Geometry check sheet. Reference: the model listing, model coordinates, mm. Face numbers are marked on the shaded views. A direction names the side the tool comes from. Give positions to 0.01 mm unless a question says otherwise; leave off trailing zeros. Order: outer loops, then holes, each group sorted by start corner. A loop starts at its lowest first (then second) coordinate and runs counter-clockwise, first axis right, second up. Notation, with made-up numbers: M 10.25,33 L 55.25,33 A31 ccw 55.25,64 Z; hole C 68,-20 d10. An arc over 180 degrees is marked long. Answer as CSV lines item,"result". Start each with the question number.
```python
from build123d import *

# Parameters (mm, degrees)
CYLINDER009_R          = 1.1
CYLINDER009_DEPTH      = 10
CYLINDER008_W          = 7
CYLINDER008_H          = 10
CYLINDER008_ANGLE      = 133
BOX008_W               = 4.5
BOX008_H               = 3.6
BOX008_DEPTH           = 10
BOX009_W               = 4.5
BOX009_H               = 3.6
BOX009_DEPTH           = 10
BOX005_W               = 3.4
BOX005_H               = 2.7
BOX005_DEPTH           = 3.5
BOX005_PLACEMENT_ANGLE = 50
BOX006_W               = 4
BOX006_H               = 2.7
BOX006_DEPTH           = 3.5
BOX006_PLACEMENT_ANGLE = 40
BOX004_W               = 3
BOX004_H               = 3
BOX004_DEPTH           = 3.5
BOX004_PLACEMENT_ANGLE = 220
BOX003_W               = 3
BOX003_H               = 3
BOX003_DEPTH           = 3.5
BOX003_PLACEMENT_ANGLE = 220
BOX001_W               = 3.4
BOX001_H               = 2.7
BOX001_DEPTH           = 3.5
BOX001_PLACEMENT_ANGLE = 50
BOX002_W               = 4
BOX002_H               = 2.7
BOX002_DEPTH           = 3.5
BOX002_PLACEMENT_ANGLE = 40
CYLINDER003_R          = 4.9
CYLINDER003_DEPTH      = 10
CYLINDER002_R          = 5.8
CYLINDER002_DEPTH      = 10
CYLINDER001_R          = 4.9
CYLINDER001_DEPTH      = 10
CYLINDER_R             = 5.7
CYLINDER_DEPTH         = 10
BOX007_W               = 38
BOX007_H               = 2
BOX007_DEPTH           = 1.5
CYLINDER004_R          = 5.95
CYLINDER004_DEPTH      = 3.5
BOX_W                  = 38
BOX_H                  = 19
BOX_DEPTH              = 2
CYLINDER005_R          = 5.95
CYLINDER005_DEPTH      = 3.5


with BuildPart() as cylinder009:
    # Cylinder009 → Cylinder009 (new body)
    with BuildSketch(Plane(origin=(13, 4.85, 0), x_dir=(1, 0, 0), z_dir=(0, 0, 1))):
        Circle(CYLINDER009_R)
    extrude(amount=CYLINDER009_DEPTH)


with BuildPart() as fusion002:
    # Cylinder008 → Cylinder008 (revolve)
    with BuildSketch(Plane(origin=(13.3, 5.5, 0), x_dir=(-1, 0, 0), z_dir=(0, 1, 0))):
        with Locations((3.5, 5)):
            Rectangle(CYLINDER008_W, CYLINDER008_H)
    revolve(axis=Axis((13.3, 5.5, 0), (0, 0, 1)), revolution_arc=CYLINDER008_ANGLE)

    # Fusion002: union Cylinder009
    add(cylinder009.part)


with BuildPart() as cube001_x_button_well_left_cutter:
    # Box008 → Box008 (new body)
    with BuildSketch(Plane(origin=(6.8, 10.2, 0.25), x_dir=(1, 0, 0), z_dir=(0, 0, 1))):
        with Locations((2.25, 1.8)):
            Rectangle(BOX008_W, BOX008_H)
    extrude(amount=BOX008_DEPTH)


with BuildPart() as cube002_y_button_well_left_cutter:
    # Box009 → Box009 (new body)
    with BuildSketch(Plane(origin=(21.1, 5.6, 0.25), x_dir=(1, 0, 0), z_dir=(0, 0, 1))):
        with Locations((2.25, 1.8)):
            Rectangle(BOX009_W, BOX009_H)
    extrude(amount=BOX009_DEPTH)


with BuildPart() as box005:
    # Box005 → Box005 (new body)
    with BuildSketch(Plane.XY):
        with Locations((1.7, 1.35)):
            Rectangle(BOX005_W, BOX005_H)
    extrude(amount=BOX005_DEPTH)


with BuildPart() as box005_1:
    # Box005 placement: moved
    add(box005.part.moved(Location((17.5, 7.5, 0.25))).rotate(Axis((17.5, 7.5, 0.25), (0, 0, -1)), BOX005_PLACEMENT_ANGLE))


with BuildPart() as box006:
    # Box006 → Box006 (new body)
    with BuildSketch(Plane.XY):
        with Locations((2, 1.35)):
            Rectangle(BOX006_W, BOX006_H)
    extrude(amount=BOX006_DEPTH)


with BuildPart() as box006_1:
    # Box006 placement: moved
    add(box006.part.moved(Location((33.7, 9, 0.25))).rotate(Axis((33.7, 9, 0.25), (0, 0, 1)), BOX006_PLACEMENT_ANGLE))


with BuildPart() as cube001_a_button_well_cutter:
    # Box004 → Box004 (new body)
    with BuildSketch(Plane.XY):
        with Locations((1.5, 1.5)):
            Rectangle(BOX004_W, BOX004_H)
    extrude(amount=BOX004_DEPTH)


with BuildPart() as cube001_a_button_well_cutter_1:
    # Box004 placement: moved
    add(cube001_a_button_well_cutter.part.moved(Location((9.8, 9.4, 0.25))).rotate(Axis((9.8, 9.4, 0.25), (0, 0, 1)), BOX004_PLACEMENT_ANGLE))


with BuildPart() as cube001_b_button_well_cutter:
    # Box003 → Box003 (new body)
    with BuildSketch(Plane.XY):
        with Locations((1.5, 1.5)):
            Rectangle(BOX003_W, BOX003_H)
    extrude(amount=BOX003_DEPTH)


with BuildPart() as cube001_b_button_well_cutter_1:
    # Box003 placement: moved
    add(cube001_b_button_well_cutter.part.moved(Location((23.5, 5, 0.25))).rotate(Axis((23.5, 5, 0.25), (0, 0, 1)), BOX003_PLACEMENT_ANGLE))


with BuildPart() as box001:
    # Box001 → Box001 (new body)
    with BuildSketch(Plane.XY):
        with Locations((1.7, 1.35)):
            Rectangle(BOX001_W, BOX001_H)
    extrude(amount=BOX001_DEPTH)


with BuildPart() as box001_1:
    # Box001 placement: moved
    add(box001.part.moved(Location((31.5, 2.9, 0.25))).rotate(Axis((31.5, 2.9, 0.25), (0, 0, -1)), BOX001_PLACEMENT_ANGLE))


with BuildPart() as cube001_y_button_well_right_top_cutter:
    # Box002 → Box002 (new body)
    with BuildSketch(Plane.XY):
        with Locations((2, 1.35)):
            Rectangle(BOX002_W, BOX002_H)
    extrude(amount=BOX002_DEPTH)


with BuildPart() as cube001_y_button_well_right_top_cutter_1:
    # Box002 placement: moved
    add(cube001_y_button_well_right_top_cutter.part.moved(Location((19.5, 13.5, 0.25))).rotate(Axis((19.5, 13.5, 0.25), (0, 0, 1)), BOX002_PLACEMENT_ANGLE))


with BuildPart() as cylinder_y_button_well_inner:
    # Cylinder003 → Cylinder003 (new body)
    with BuildSketch(Plane(origin=(29.55, 7.35, 0), x_dir=(1, 0, 0), z_dir=(0, 0, 1))):
        Circle(CYLINDER003_R)
    extrude(amount=CYLINDER003_DEPTH)


with BuildPart() as cylinder_b_button_well_inner:
    # Cylinder002 → Cylinder002 (new body)
    with BuildSketch(Plane(origin=(18.7, -1.6, 0), x_dir=(1, 0, 0), z_dir=(0, 0, 1))):
        Circle(CYLINDER002_R)
    extrude(amount=CYLINDER002_DEPTH)


with BuildPart() as cylinder_x_button_well_inner:
    # Cylinder001 → Cylinder001 (new body)
    with BuildSketch(Plane(origin=(15.55, 11.7, 0), x_dir=(1, 0, 0), z_dir=(0, 0, 1))):
        Circle(CYLINDER001_R)
    extrude(amount=CYLINDER001_DEPTH)


with BuildPart() as cylinder_a_button_well_inner:
    # Cylinder → Cylinder (new body)
    with BuildSketch(Plane(origin=(4.6, 3.2, 0), x_dir=(1, 0, 0), z_dir=(0, 0, 1))):
        Circle(CYLINDER_R)
    extrude(amount=CYLINDER_DEPTH)


with BuildPart() as fusion001:
    # Box007 → Box007 (new body)
    with BuildSketch(Plane(origin=(0, 18, 0), x_dir=(1, 0, 0), z_dir=(0, 0, 1))):
        with Locations((19, 1)):
            Rectangle(BOX007_W, BOX007_H)
    extrude(amount=BOX007_DEPTH)

    # Fusion001: union Cube001(x_button_well_left_cutter), Cube002(y_button_well_left_cutter), Box005, Box006, Cube001(a_button_well_cutter), Cube001(b_button_well_cutter), Box001, Cube001(y_button_well_right_top_cutter), Cylinder(y_button_well_inner), Cylinder(b_button_well_inner), Cylinder(x_button_well_inner), Cylinder(a_button_well_inner)
    add(cube001_x_button_well_left_cutter.part)
    add(cube002_y_button_well_left_cutter.part)
    add(box005_1.part)
    add(box006_1.part)
    add(cube001_a_button_well_cutter_1.part)
    add(cube001_b_button_well_cutter_1.part)
    add(box001_1.part)
    add(cube001_y_button_well_right_top_cutter_1.part)
    add(cylinder_y_button_well_inner.part)
    add(cylinder_b_button_well_inner.part)
    add(cylinder_x_button_well_inner.part)
    add(cylinder_a_button_well_inner.part)


with BuildPart() as cylinder_x_button_well_outer:
    # Cylinder004 → Cylinder004 (new body)
    with BuildSketch(Plane(origin=(15.55, 11.7, 0), x_dir=(1, 0, 0), z_dir=(0, 0, 1))):
        Circle(CYLINDER004_R)
    extrude(amount=CYLINDER004_DEPTH)


with BuildPart() as cube:
    # Box → Box (new body)
    with BuildSketch(Plane.XY):
        with Locations((19, 9.5)):
            Rectangle(BOX_W, BOX_H)
    extrude(amount=BOX_DEPTH)


with BuildPart() as cut001:
    # Cylinder005 → Cylinder005 (new body)
    with BuildSketch(Plane(origin=(29.55, 7.35, 0), x_dir=(1, 0, 0), z_dir=(0, 0, 1))):
        Circle(CYLINDER005_R)
    extrude(amount=CYLINDER005_DEPTH)

    # Fusion: union Cylinder(x_button_well_outer), Cube
    add(cylinder_x_button_well_outer.part)
    add(cube.part)

    # Cut: cut Fusion001
    add(fusion001.part, mode=Mode.SUBTRACT)

    # Cut001: cut Fusion002
    add(fusion002.part, mode=Mode.SUBTRACT)


solid = cut001.part
```
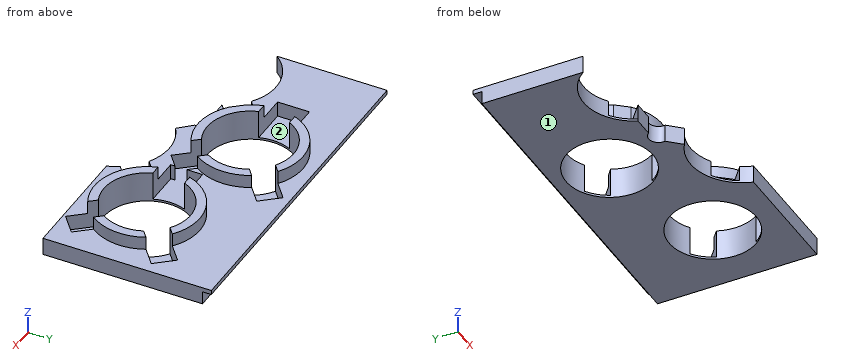
Item 1: Scan lines: line 1 along X through (y, z) = (7.35, 0.7); line 2 along X through (y, z) = (11.5, 1.65); line 3 along X through (y, z) = (5.75, 1.45). Record each from-to range of solid material in increasing order.
Item 2: Section check D-D on x = 4. Record the boundary of the cut face in (y, z).
Item 3: Section check C-C on x = 8.5. Record the boundary of the cut face in (y, z).
Item 4: Depth check by flat-ended pin: pin 1 Ø0.8 at (x, z) = (20, 1) entering from +Y; pin 2 Ø1.5 at (x, z) = (15.5, 3) entering from +Y; pin 3 Ø1.3 at (x, y) = (21.5, 6.5) entering from +Z. Enter the tip coordinate at first touch or a pass-through.
Item 5: Section check A-A on x = 29.55. Record the boundary of the cut face in (y, z).
Item 6: Section check B-B on z = 3. Record the boundary of the cut face in (x, y), then the cut area to 3 significant figures.
Item 7: Access from +Z, -Z, +X, -X, +Y, -Y to the whole of each face (thin tool, end or side, straight path). Record for the marked faces 1 and 2.
Numbers:
1,line 1,"0 to 0.69, 11.52 to 13.29, 34.45 to 38"
1,line 2,"0 to 6.8, 20.45 to 26.94, 32.16 to 32.48, 36.68 to 38"
1,line 3,"10.12 to 12.37, 13.63 to 18.97, 20.7 to 21.1, 34.18 to 38"
2,outline,"M 8.87,0 L 18,0 L 18,1.5 L 19,1.5 L 19,2 L 8.87,2 Z"
3,outline,"M 7.36,0 L 18,0 L 18,1.5 L 19,1.5 L 19,2 L 13.8,2 L 13.8,0.25 L 10.2,0.25 L 10.2,2 L 8.31,2 L 8.31,0.25 L 7.36,0.25 Z"
4,pin 1,"y = 18"
4,pin 2,"y = 17.65"
4,pin 3,"z = 2"
5,outline,"M 0,0 L 2.45,0 L 2.45,3.5 L 1.4,3.5 L 1.4,2 L 0,2 Z; M 12.25,0 L 18,0 L 18,1.5 L 19,1.5 L 19,2 L 13.3,2 L 13.3,3.5 L 12.25,3.5 Z"
6,outline,"M 9.79,10.2 A5.95 ccw 10.47,8.6 L 11.61,7.24 A5.95 ccw 18.37,6.46 L 17.68,7.29 A4.9 cw 10.89,10.2 Z; M 9.98,13.8 L 11.12,13.8 A4.9 cw 18.12,15.87 L 18.96,16.57 A5.95 ccw Z; M 19.69,9.09 L 20.4,8.25 A5.95 ccw 20.77,14.56 L 19.94,13.87 A4.9 cw Z; M 23.86,5.6 A5.95 ccw 32.23,2.04 L 31.53,2.87 A4.9 cw 24.97,5.6 Z; M 23.89,9.2 L 25.01,9.2 A4.9 cw 32.34,11.38 L 33.17,12.08 A5.95 ccw Z; M 33.6,4.6 L 34.3,3.77 A5.95 ccw 34.88,9.99 L 34.05,9.29 A4.9 cw Z"
6,area,"52.3 mm2"
7,face 1,"-Z, +X, -X, +Y, -Y"
7,face 2,"+Z"
